```python
from build123d import *

# Parameters (mm, degrees)
CROQUIS1_R              = 2.5
CROQUIS1_R_2            = 14.25
SALIENTE_EXTRUIR1_DEPTH = 3
CROQUIS3_W              = 3
CROQUIS3_H              = 13.002457907
CROQUIS3_H_2            = 13.048194377
CROQUIS3_H_3            = 13.048194378
CORTAR_EXTRUIR1_DEPTH   = 3
CROQUIS4_W              = 163.675423661
CROQUIS4_H              = 10
CORTAR_EXTRUIR2_DEPTH   = 10
REDONDEO1_R             = 10
CROQUIS5_R              = 2.5
CORTAR_EXTRUIR3_DEPTH   = 10
CORTAR_EXTRUIR4_DEPTH   = 10
CORTAR_EXTRUIR5_DEPTH   = 10
REDONDEO2_R             = 10


with BuildPart() as part:
    # Croquis1 → Saliente-Extruir1 (new body)
    with BuildSketch(Plane.XY):
        with BuildLine():
            Line((-135.811178416, 31.660861846), (-65.873242367, 31.660861846))
            ThreePointArc((-65.873242367, 31.660861846), (-63.837291884, 32.094144685), (-62.154198363, 33.318899594))
            Line((-62.154198363, 33.318899594), (39.377470593, 146.306634388))
            ThreePointArc((39.377470593, 146.306634388), (43.719655801, 147.925689677), (47.526539972, 145.28304984))
            Line((47.526539972, 145.28304984), (132.635412267, -17.345525839))
            ThreePointArc((132.635412267, -17.345525839), (124.188821584, -44.339138154), (97.195209269, -35.892547471))
            Line((97.195209269, -35.892547471), (38.788084081, 75.713532162))
            ThreePointArc((38.788084081, 75.713532162), (34.981199909, 78.356171999), (30.639014702, 76.737116711))
            Line((30.639014702, 76.737116711), (-44.321252629, -6.681100406))
            ThreePointArc((-44.321252629, -6.681100406), (-46.00434615, -7.905855315), (-48.040296633, -8.339138154))
            Line((-48.040296633, -8.339138154), (-135.811178416, -8.339138154))
            ThreePointArc((-135.811178416, -8.339138154), (-155.811178416, 11.660861846), (-135.811178416, 31.660861846))
        make_face()
        with Locations((-135.811178416, 11.660861846)):
            Circle(CROQUIS1_R, mode=Mode.SUBTRACT)
        with Locations((-65.81121578, 11.5885363)):
            Circle(CROQUIS1_R, mode=Mode.SUBTRACT)
        with Locations((109.098617172, -15.504324767)):
            Circle(CROQUIS1_R_2, mode=Mode.SUBTRACT)
    extrude(amount=SALIENTE_EXTRUIR1_DEPTH)

    # Croquis3 → Cortar-Extruir1 (cut)
    with BuildSketch(Plane(origin=(96.993591322, 50.759930368, 0), x_dir=(0, 0, -1), z_dir=(0.8860050749641628, 0.46367554080169926, 0))):
        with Locations((-1.5, 79.927636726)):
            Rectangle(CROQUIS3_W, CROQUIS3_H)
        with Locations((-1.5, 49.42886568)):
            Rectangle(CROQUIS3_W, CROQUIS3_H_2)
        with Locations((-1.5, 18.952962868)):
            Rectangle(CROQUIS3_W, CROQUIS3_H_3)
    extrude(amount=-CORTAR_EXTRUIR1_DEPTH, mode=Mode.SUBTRACT)

    # Croquis4 → Cortar-Extruir2 (cut)
    with BuildSketch(Plane.XY.offset(3)):
        with Locations((-95.362453556, -3.339138154)):
            Rectangle(CROQUIS4_W, CROQUIS4_H)
    extrude(amount=-CORTAR_EXTRUIR2_DEPTH, mode=Mode.SUBTRACT)

    # Redondeo1
    redondeo1_edges = [part.edges().sort_by_distance(p)[0] for p in [
        (-153.131686492, 1.660861846, 1.5),
        (-36.825099605, 1.660861846, 1.5),
    ]]
    fillet(redondeo1_edges, radius=REDONDEO1_R)

    # Croquis5 → Cortar-Extruir3 (cut)
    with BuildSketch(Plane.XY.offset(3)):
        Polygon((-63.64412415, 31.660861846), (-72.924071867, 21.333834995), (-57.92427468, 21.255832735), (-48.581088821, 31.660861846), align=None)
        Polygon((-62.154198363, 33.318899594), (-63.64412415, 31.660861846), (-48.581088821, 31.660861846), (37.330618128, 127.336343983), (22.330618128, 127.336343983), align=None)
        with Locations((-100.811197098, 11.624699073)):
            Circle(CROQUIS5_R)
    extrude(amount=-CORTAR_EXTRUIR3_DEPTH, mode=Mode.SUBTRACT)

    # Croquis6 → Cortar-Extruir4 (cut)
    with BuildSketch(Plane.XY.offset(3)):
        Polygon((-72.924071867, 21.333834995), (-60.713701646, 34.921931069), (-169.534972591, 34.921931069), (-169.534972591, 0), (-115.124337118, 0), (-115.124337118, 21.333834995), align=None)
    extrude(amount=-CORTAR_EXTRUIR4_DEPTH, mode=Mode.SUBTRACT)

    # Croquis7 → Cortar-Extruir5 (cut)
    with BuildSketch(Plane.XY.offset(3)):
        Polygon((22.330618128, 127.336343983), (78.839367292, 127.336343983), (43.163788292, 161.798984153), align=None)
    extrude(amount=-CORTAR_EXTRUIR5_DEPTH, mode=Mode.SUBTRACT)

    # Redondeo2
    # the kernel refuses this fillet: 10 mm, written as the material it adds along each edge
    with BuildSketch(Plane(origin=(-57.92427468, 21.255832735, 3), x_dir=(0.6681211936204373, 0.744052464974885, 0), z_dir=(0, 0, -1))) as redondeo2_piece_1:
        with BuildLine():
            CenterArc((REDONDEO2_R * 0.449163221223, -REDONDEO2_R), REDONDEO2_R, 90, 48.37572531)
            Line((-REDONDEO2_R * 0.298353514379, -REDONDEO2_R * 0.335757024882), (0, 0))
            Line((0, 0), (REDONDEO2_R * 0.449163221223, 0))
        make_face()
    extrude(amount=3)
    # the kernel refuses this fillet: 10 mm, written as the material it takes off along each edge
    with BuildSketch(Plane(origin=(-115.124337118, 1.660861846, 28), x_dir=(1, 0, 0), z_dir=(0, 0, -1))) as redondeo2_2_piece_1:
        with BuildLine():
            CenterArc((REDONDEO2_R, -REDONDEO2_R), REDONDEO2_R, 90, 90)
            Line((0, -REDONDEO2_R), (0, 0))
            Line((0, 0), (REDONDEO2_R, 0))
        make_face()
    extrude(amount=53, mode=Mode.SUBTRACT)
    with BuildSketch(Plane(origin=(-115.124337118, 21.333834995, 28), x_dir=(1, 0, 0), z_dir=(0, 0, -1))) as redondeo2_2_piece_2:
        with BuildLine():
            CenterArc((REDONDEO2_R, REDONDEO2_R), REDONDEO2_R, 180, 90)
            Line((0, REDONDEO2_R), (0, 0))
            Line((0, 0), (REDONDEO2_R, 0))
        make_face()
    extrude(amount=53, mode=Mode.SUBTRACT)


solid = part.part
```
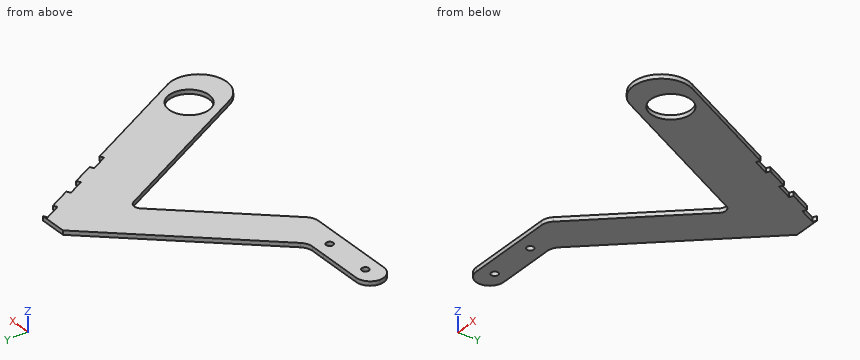
Geometry: final body of the model. Coordinates: model frame, mm. Give positions to 0.01 mm unless a question says otherwise; leave off trailing zeros. Write each loop counter-clockwise with the first axis right and the second up, starting at its lowest first coordinate (ties: lowest second). Pieces come first, ordered by that corner, then holes.
1. Section query A-A, the plane y = 46. Return loops of the section in (x, z), then the cut area to 3 significant figures.
2. Section query C-C, the plane y = 68.5. Return loops of the section in (x, z), then the cut area to 3 significant figures.
3. Line query: probe 1 along X at (y, z) = (-9, 2.7); probe 2 along X at (y, z) = (49.5, 1.6); probe 3 along Y at (x, z) = (-80, 2.15). Output: solid intervals per line, ascending.
4. Section query B-B, the plane z = 1.45. Return loops of the section in (x, y).
5. Pin query (flat end, axial travel): P1, Ø1.5, axis at y = -25, z = 2.5, coming from the -X side; P2, Ø0.9, axis at x = -92.5, z = 1, coming from the +Y side. Return the tip coordinate at first contact, or that it passes through.
6. Section query D-D, the plane x = 3.5. Return loops of the section in (y, z).
Computed:
1. outline: (-35.71, 0) - (3.02, 0) - (3.02, 3) - (-35.71, 3) - close; (54.34, 0) - (99.48, 0) - (99.48, 3) - (54.34, 3) - close
1. area: 252 mm2
2. outline: (-15.5, 0) - (23.24, 0) - (23.24, 3) - (-15.5, 3) - close; (42.56, 0) - (84.32, 0) - (84.32, 3) - (42.56, 3) - close
2. area: 241 mm2
3. probe 1: x = 83.12 to 96.42, 121.78 to 128.27
3. probe 2: x = -32.56 to 6.16, 52.51 to 97.65
3. probe 3: y = 1.66 to 21.33
4. outline: (-115.12, 11.5) arc R10 ccw to (-105.12, 1.66) - (-41.28, 1.66) arc R10 ccw to (-33.85, 4.98) - (30.64, 76.74) arc R5 cw to (38.79, 75.71) - (97.2, -35.89) arc R20 ccw to (132.64, -17.35) - (91.23, 61.77) - (88.57, 60.38) - (82.52, 71.94) - (85.18, 73.33) - (77.1, 88.77) - (74.44, 87.38) - (68.39, 98.94) - (71.05, 100.33) - (62.95, 115.82) - (60.29, 114.43) - (54.26, 125.95) - (56.92, 127.34) - (37.33, 127.34) - (-54.92, 24.6) arc R10 cw to (-62.42, 21.28) - (-72.92, 21.33) - (-105.12, 21.33) arc R10 ccw to start; hole circle Ø5 at (-100.81, 11.62); hole circle Ø5 at (-65.81, 11.59); hole circle Ø28.5 at (109.1, -15.5)
5. P1: stops at x = 91.1
5. P2: stops at y = 21.33
6. outline: (46.54, 0) - (89.66, 0) - (89.66, 3) - (46.54, 3) - close
